```python
from build123d import *

# Parameters (mm, degrees)
SKETCH_1_W      = 41
SKETCH_1_H      = 16
SKETCH_1_R      = 2
EXTRUDE_1_DEPTH = 2
FILLET_1_R      = 1
FILLET_2_R      = 1
FILLET_3_R      = 1
FILLET_4_R      = 1


with BuildPart() as part:
    # 草图1 → 凸台-拉伸1 (new body)
    with BuildSketch(Plane(origin=(0, 0, 0), x_dir=(1, 0, 0), z_dir=(0, 1, 0))):
        Rectangle(SKETCH_1_W, SKETCH_1_H)
        with Locations(Location((-14, 0, 0), (0, 0, 270))):
            Circle(SKETCH_1_R, mode=Mode.SUBTRACT)
        with Locations(Location((14, 0, 0), (0, 0, 90))):
            Circle(SKETCH_1_R, mode=Mode.SUBTRACT)
    extrude(amount=EXTRUDE_1_DEPTH)

    # 圆角1
    fillet_1_edges = [part.edges().sort_by_distance(p)[0] for p in [
        (20.5, 1, 8),
    ]]
    fillet(fillet_1_edges, radius=FILLET_1_R)

    # 圆角2
    fillet_2_edges = [part.edges().sort_by_distance(p)[0] for p in [
        (-20.5, 1, 8),
    ]]
    fillet(fillet_2_edges, radius=FILLET_2_R)

    # 圆角3
    fillet_3_edges = [part.edges().sort_by_distance(p)[0] for p in [
        (-20.5, 1, -8),
    ]]
    fillet(fillet_3_edges, radius=FILLET_3_R)

    # 圆角4
    fillet_4_edges = [part.edges().sort_by_distance(p)[0] for p in [
        (20.5, 1, -8),
    ]]
    fillet(fillet_4_edges, radius=FILLET_4_R)


solid = part.part
```
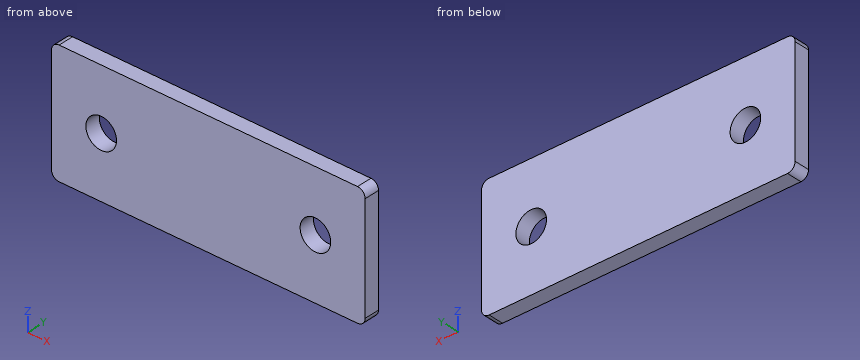
Check sheet for the modelled part. Datum: model origin and axes. Units: mm. Give positions to 0.01 mm unless a question says otherwise; leave off trailing zeros. Loops run counter-clockwise (first coordinate to the right, second up) from the corner with the lowest first, then second, coordinate; pieces in that order, holes last. Notation, with made-up numbers: M 72.25,75.25 L 101.25,75.25 A27 cw 101.25,110.25 Z; hole C -32.75,-5.75 d1. An arc over 180 degrees is marked long. Answer as CSV lines item,"result".
Item 1: Sectioned sample at A-A, the plane x = -14. Enter the section's corners in (y, z), then the cut area to 3 significant figures.
Reply:
outline,"M 0,-8 L 2,-8 L 2,-2 L 0,-2 Z; M 0,2 L 2,2 L 2,8 L 0,8 Z"
area,"24.0 mm^2"
Item 2: Sectioned sample at B-B, the plane z = 0. Enter the section's corners in (x, y), then the cut area to 3 significant figures.
Reply:
outline,"M -20.5,0 L -16,0 L -16,2 L -20.5,2 Z; M -12,0 L 12,0 L 12,2 L -12,2 Z; M 16,0 L 20.5,0 L 20.5,2 L 16,2 Z"
area,"66.0 mm^2"
Item 3: Scan lines: L1, parallel to X at y = 0.85, z = 0; L2, parallel to Z at x = 14, y = 0.4; L3, parallel to X at y = 0.9, z = -0.5. Record each from-to range of solid material in increasing order.
Reply:
L1,"-20.5 to -16, -12 to 12, 16 to 20.5"
L2,"-8 to -2, 2 to 8"
L3,"-20.5 to -15.94, -12.06 to 12.06, 15.94 to 20.5"
Item 4: Sectioned sample at C-C, the plane y = 0.95. Enter the section's corners in (x, z).
Reply:
outline,"M -20.5,-7 A1 ccw -19.5,-8 L 19.5,-8 A1 ccw 20.5,-7 L 20.5,7 A1 ccw 19.5,8 L -19.5,8 A1 ccw -20.5,7 Z; hole C -14,0 d4; hole C 14,0 d4"
